Verification items for the finished model (mm, model axes). Face numbers are marked on the shaded views. A direction names the side the tool comes from. Give positions to 0.01 mm unless a question says otherwise; leave off trailing zeros. Order: outer loops, then holes, each group sorted by start corner. A loop starts at its lowest first (then second) coordinate and runs counter-clockwise, first axis right, second up.
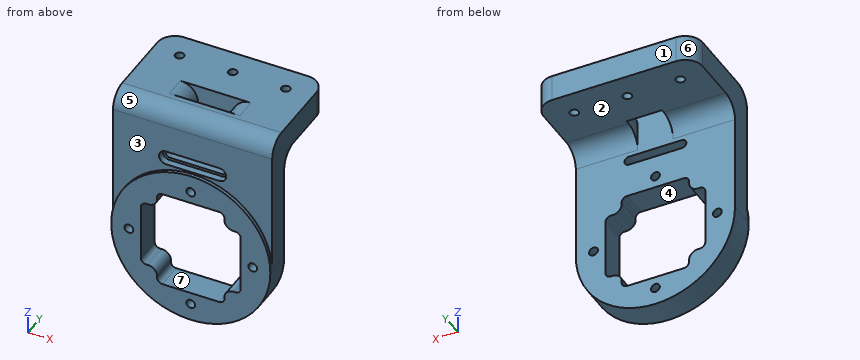
from build123d import *

# Parameters (mm, degrees)
BOSS_EXTRUDE1_DEPTH     = 15
SKETCH2_W               = 90
SKETCH2_H               = 15
BOSS_EXTRUDE2_DEPTH     = 45
CUT_EXTRUDE1_DEPTH      = 2
SKETCH4_R               = 2.5
CUT_EXTRUDE2_DEPTH      = 110.658560997
FILLET1_R               = 10
SKETCH5_R               = 2.5
CUT_EXTRUDE3_DEPTH      = 134.135269557
CUT_EXTRUDE4_DEPTH      = 103.225241501
CUT_EXTRUDE5_DEPTH      = 4
CUT_EXTRUDE6_DEPTH      = 10
CUT_EXTRUDE6_DEPTH_BACK = 15
SKETCH8_W               = 20
SKETCH8_H               = 12
FILLET2_R               = 10


with BuildPart() as part:
    # Sketch1 → Boss-Extrude1 (new body)
    with BuildSketch(Plane(origin=(0, 0, 0), x_dir=(1, 0, 0), z_dir=(0, 1, 0))):
        with BuildLine():
            ThreePointArc((45, 0), (0, -45), (-45, 0))
            Line((-45, 0), (-45, -80))
            Line((-45, -80), (45, -80))
            Line((45, -80), (45, 0))
        make_face()
        with BuildLine():
            Line((-28.2, -16.05), (-28.2, 0))
            Line((-28.2, 0), (-45, 0))
            ThreePointArc((-45, 0), (0, -45), (45, 0))
            Line((45, 0), (28.2, 0))
            Line((28.2, 0), (28.2, -16.05))
            ThreePointArc((28.2, -16.05), (27.321320344, -18.171320344), (25.2, -19.05))
            Line((25.2, -19.05), (24.05, -19.05))
            ThreePointArc((24.05, -19.05), (20.514466094, -20.514466094), (19.05, -24.05))
            Line((19.05, -24.05), (19.05, -25.2))
            ThreePointArc((19.05, -25.2), (18.171320344, -27.321320344), (16.05, -28.2))
            Line((16.05, -28.2), (-16.05, -28.2))
            ThreePointArc((-16.05, -28.2), (-18.171320344, -27.321320344), (-19.05, -25.2))
            Line((-19.05, -25.2), (-19.05, -24.05))
            ThreePointArc((-19.05, -24.05), (-20.514466094, -20.514466094), (-24.05, -19.05))
            Line((-24.05, -19.05), (-25.2, -19.05))
            ThreePointArc((-25.2, -19.05), (-27.321320344, -18.171320344), (-28.2, -16.05))
        make_face()
        with BuildLine():
            ThreePointArc((-19.05, 25.2), (-18.171320344, 27.321320344), (-16.05, 28.2))
            Line((-16.05, 28.2), (16.05, 28.2))
            ThreePointArc((16.05, 28.2), (18.171320344, 27.321320344), (19.05, 25.2))
            Line((19.05, 25.2), (19.05, 24.05))
            ThreePointArc((19.05, 24.05), (20.514466094, 20.514466094), (24.05, 19.05))
            Line((24.05, 19.05), (25.2, 19.05))
            ThreePointArc((25.2, 19.05), (27.321320344, 18.171320344), (28.2, 16.05))
            Line((28.2, 16.05), (28.2, 0))
            Line((28.2, 0), (45, 0))
            ThreePointArc((45, 0), (0, 45), (-45, 0))
            Line((-45, 0), (-28.2, 0))
            Line((-28.2, 0), (-28.2, 16.05))
            ThreePointArc((-28.2, 16.05), (-27.321320344, 18.171320344), (-25.2, 19.05))
            Line((-25.2, 19.05), (-24.05, 19.05))
            ThreePointArc((-24.05, 19.05), (-20.514466094, 20.514466094), (-19.05, 24.05))
            Line((-19.05, 24.05), (-19.05, 25.2))
        make_face()
    extrude(amount=BOSS_EXTRUDE1_DEPTH)

    # Sketch2 → Boss-Extrude2 (add)
    with BuildSketch(Plane(origin=(0, 15, 0), x_dir=(1, 0, 0), z_dir=(0, 1, 0))):
        with Locations((0, -72.5)):
            Rectangle(SKETCH2_W, SKETCH2_H)
    extrude(amount=BOSS_EXTRUDE2_DEPTH)

    # Sketch3 → Cut-Extrude1 (cut)
    with BuildSketch(Plane(origin=(0, 0, 0), x_dir=(-1, 0, 0), z_dir=(0, -1, 0))):
        with BuildLine():
            Line((45, -80), (-45, -80))
            Line((-45, -80), (-45, 0))
            ThreePointArc((-45, 0), (0, -45), (45, 0))
            Line((45, 0), (45, -80))
        make_face()
    extrude(amount=-CUT_EXTRUDE1_DEPTH, mode=Mode.SUBTRACT)

    # Sketch4 → Cut-Extrude2 (cut, through all)
    with BuildSketch(Plane(origin=(0, 0, 0), x_dir=(-1, 0, 0), z_dir=(0, -1, 0))):
        with Locations(Location((0, -35, 0), (0, 0, 90))):
            Circle(SKETCH4_R)
        with Locations(Location((-35, 0, 0), (0, 0, 90))):
            Circle(SKETCH4_R)
        with Locations(Location((0, 35, 0), (0, 0, 90))):
            Circle(SKETCH4_R)
        with Locations(Location((35, 0, 0), (0, 0, 90))):
            Circle(SKETCH4_R)
    extrude(amount=-CUT_EXTRUDE2_DEPTH, mode=Mode.SUBTRACT)

    # Fillet1
    fillet1_edges = [part.edges().sort_by_distance(p)[0] for p in [
        (0, 2, 80),
        (-45, 60, 72.5),
        (45, 60, 72.5),
        (0, 15, 65),
    ]]
    fillet(fillet1_edges, radius=FILLET1_R)

    # Sketch5 → Cut-Extrude3 (cut, through all)
    with BuildSketch(Plane(origin=(0, 0, 65), x_dir=(-1, 0, 0), z_dir=(0, 0, -1))):
        with Locations((-30, 45.502937017)):
            Circle(SKETCH5_R)
        with Locations((30, 45.502937017)):
            Circle(SKETCH5_R)
        with Locations((0, 45.502937017)):
            Circle(SKETCH5_R)
    extrude(amount=-CUT_EXTRUDE3_DEPTH, mode=Mode.SUBTRACT)

    # Sketch6 → Cut-Extrude4 (cut, through all)
    with BuildSketch(Plane(origin=(0, 15, 0), x_dir=(1, 0, 0), z_dir=(0, 1, 0))):
        with BuildLine():
            Line((-15, -47.5), (15, -47.5))
            ThreePointArc((15, -47.5), (17.5, -50), (15, -52.5))
            Line((15, -52.5), (-15, -52.5))
            ThreePointArc((-15, -52.5), (-17.5, -50), (-15, -47.5))
        make_face()
    extrude(amount=-CUT_EXTRUDE4_DEPTH, mode=Mode.SUBTRACT)

    # Sketch7 → Cut-Extrude5 (cut)
    with BuildSketch(Plane.XZ.offset(-2)):
        with BuildLine():
            Line((-15, 54), (15, 54))
            ThreePointArc((15, 54), (19, 50), (15, 46))
            Line((15, 46), (-15, 46))
            ThreePointArc((-15, 46), (-19, 50), (-15, 54))
        make_face()
    extrude(amount=-CUT_EXTRUDE5_DEPTH, mode=Mode.SUBTRACT)

    # Sketch8 → Cut-Extrude6 (cut, two sides: drawn at the far end of the back side and taken through both)
    with BuildSketch(Plane(origin=(0, 0, 65), x_dir=(-1, 0, 0), z_dir=(0, 0, -1)).offset(-CUT_EXTRUDE6_DEPTH_BACK)):
        with Locations((0, 21)):
            Rectangle(SKETCH8_W, SKETCH8_H)
    extrude(amount=CUT_EXTRUDE6_DEPTH + CUT_EXTRUDE6_DEPTH_BACK, mode=Mode.SUBTRACT)

    # Fillet2
    fillet2_edges = [part.edges().sort_by_distance(p)[0] for p in [
        (10, 21, 80),
        (-10, 21, 80),
    ]]
    fillet(fillet2_edges, radius=FILLET2_R)


solid = part.part
(1) Section check D-D, the plane y = 8.5. Give the number of separate pieces and of enclosed holes in the cut face, then the cut area to 3 significant figures.
Solved:
separate pieces: 1
enclosed holes: 6
area: 7,220 mm2
(2) Section check C-C, the plane x = 30. Enter the section's corners in (y, z), then the cut area to 3 significant figures.
Solved:
outline: (0, -33.54) - (15, -33.54) - (15, 55) arc R10 cw to (25, 65) - (43, 65) - (43, 80) - (12, 80) arc R10 ccw to (2, 70) - (2, 33.54) - (0, 33.54) - close; (48, 65) - (60, 65) - (60, 80) - (48, 80) - close
area: 2,210 mm2
(3) Section check B-B, the plane x = -6.5. Enter the section's corners in (y, z).
Solved:
outline: (0, -44.53) - (15, -44.53) - (15, -28.2) - (0, -28.2) - close; (0, 28.2) - (15, 28.2) - (15, 47.5) - (6, 47.5) - (6, 46) - (2, 46) - (2, 44.53) - (0, 44.53) - close; (2, 54) - (6, 54) - (6, 52.5) - (15, 52.5) - (15, 80) - (12, 80) arc R10 ccw to (2, 70) - close; (27, 65) - (60, 65) - (60, 80) - (27, 80) - close
(4) Set-up check for the marked faces 1, 2 and 3: record each of +Z, -Z, +X, -X, +Y, -Y from which the full face is reachable in a straight line by a thin tool's end or side.
Solved:
face 1: +Z, -Z, +X, -X, +Y
face 2: -Z, +X, -X, +Y
face 3: +Z, -Y
(5) Section check A-A, the plane z = 50. Enter the section's corners in (x, y).
Solved:
outline: (-45, 2) - (-19, 2) - (-19, 6) - (-17.5, 6) - (-17.5, 15) - (-45, 15) - close; (17.5, 6) - (19, 6) - (19, 2) - (45, 2) - (45, 15) - (17.5, 15) - close
(6) Release check for a two-part mould opening along Z. For the marked faces 4, 5, 6 and 7 record: pulls with the +Z half, pulls with the -Z half, needs draft (parallel to the pull), parting line crosses it, or undercut.
Solved:
face 4: undercut
face 5: pulls with the +Z half
face 6: needs draft
face 7: undercut
(7) Scan lines: line 1 (X direction, y = 21.5, z = 64.5); line 2 (Y direction, x = 30, z = 68.25); line 3 (X direction, y = 44.5, z = 70). Record each from-to range of solid material in increasing order.
Solved:
line 1: x = -45 to -10, 10 to 45
line 2: y = 2 to 43, 48 to 60
line 3: x = -45 to -32.29, -27.71 to -2.29, 2.29 to 27.71, 32.29 to 45
(8) Go/stop test with flat-tipped pins: pin 1 (16.5 mm diameter, centred on x = -6.5, z = 71, fed in from -Y); pin 2 (0.6 mm diameter, centred on y = 11, z = -25, fed in from +X); pin 3 (0.6 mm diameter, centred on x = -24.5, y = 10, fed in from -Z); pin 4 (4.5 mm diameter, centred on x = 0, y = 45.5, fed in from +Z). Record where each tip stops, or that it passes through.
Solved:
pin 1: stops at y = 2
pin 2: stops at x = 37.62
pin 3: stops at z = -37.94
pin 4: passes through
